from build123d import *

# Parameters (mm, degrees)
SKETCH_1_R               = 2.2
EXTRUDE_2_DEPTH          = 4
SKETCH_2_W               = 4
SKETCH_2_H               = 25
EXTRUDE_3_DEPTH          = 16
SKETCH_3_W               = 4
SKETCH_3_H               = 25
EXTRUDE_4_DEPTH          = 50
SKETCH_4_W               = 18
SKETCH_4_H               = 6.5
EXTRUDE_5_DEPTH          = 4
SKETCH_5_W               = 18
SKETCH_5_H               = 4
EXTRUDE_6_DEPTH          = 5
SKETCH_6_W               = 2.5
SKETCH_6_H               = 4
SKETCH_6_W_2             = 3
SKETCH_6_H_2             = 18
CUT_EXTRUDE_1_DEPTH      = 4
CUT_EXTRUDE_2_DEPTH      = 64.095166217
CUT_EXTRUDE_2_DEPTH_BACK = 64.095166217
SKETCH_7_R               = 4.7
CUT_EXTRUDE_3_DEPTH      = 64.095166217
EXTRUDE_7_DEPTH          = 3
EXTRUDE_8_DEPTH          = 3
CHAMFER_1_SIZE           = 3
CHAMFER_2_SIZE           = 2
FILLET_1_R               = 3
SKETCH_11_W              = 18
SKETCH_11_H              = 1
CUT_EXTRUDE_4_DEPTH      = 10
FILLET_2_R               = 2


with BuildPart() as part:
    # 草图1 → 凸台-拉伸2 (new body)
    with BuildSketch(Plane.XY):
        Polygon((0, 35), (0, 10), (-2.83, 10), (-2.83, 0), (9.32, 0), (9.32, 35), align=None)
        with Locations((2.17, 5)):
            Circle(SKETCH_1_R, mode=Mode.SUBTRACT)
        with Locations((5.17, 30)):
            Circle(SKETCH_1_R, mode=Mode.SUBTRACT)
    extrude(amount=EXTRUDE_2_DEPTH)

    # 草图2 → 凸台-拉伸3 (add)
    with BuildSketch(Plane(origin=(0, 0, 0), x_dir=(-1, 0, 0), z_dir=(0, 0, -1))):
        with Locations((2, 22.5)):
            Rectangle(SKETCH_2_W, SKETCH_2_H)
    extrude(amount=-EXTRUDE_3_DEPTH)

    # 草图3 → 凸台-拉伸4 (add)
    with BuildSketch(Plane(origin=(0, 0, 0), x_dir=(0, 0, -1), z_dir=(1, 0, 0))):
        with Locations((-14, 22.5)):
            Rectangle(SKETCH_3_W, SKETCH_3_H)
    extrude(amount=-EXTRUDE_4_DEPTH)

    # 草图4 → 凸台-拉伸5 (add)
    with BuildSketch(Plane(origin=(0, 0, 12), x_dir=(-1, 0, 0), z_dir=(0, 0, -1))):
        with Locations((33, 6.75)):
            Rectangle(SKETCH_4_W, SKETCH_4_H)
    extrude(amount=-EXTRUDE_5_DEPTH)

    # 草图5 → 凸台-拉伸6 (add)
    with BuildSketch(Plane(origin=(0, 0, 12), x_dir=(-1, 0, 0), z_dir=(0, 0, -1))):
        with Locations((33, 5.5)):
            Rectangle(SKETCH_5_W, SKETCH_5_H)
        with Locations((33, 33)):
            Rectangle(SKETCH_5_W, SKETCH_5_H)
    extrude(amount=EXTRUDE_6_DEPTH)

    # 草图6 → 切除-拉伸1 (cut)
    with BuildSketch(Plane(origin=(0, 0, 12), x_dir=(-1, 0, 0), z_dir=(0, 0, -1))):
        with Locations((15.05, 12)):
            Rectangle(SKETCH_6_W, SKETCH_6_H)
        with Locations((48.5, 19)):
            Rectangle(SKETCH_6_W_2, SKETCH_6_H_2)
    extrude(amount=-CUT_EXTRUDE_1_DEPTH, mode=Mode.SUBTRACT)

    # 草图7 → 切除-拉伸2 (cut, two sides: drawn at the far end of the back side and taken through both)
    with BuildSketch(Plane(origin=(0, 0, 0), x_dir=(0, 0, -1), z_dir=(1, 0, 0)).offset(-CUT_EXTRUDE_2_DEPTH_BACK)):
        with Locations(Location((-7.3, 20, 0), (0, 0, 45.402043339))):
            Circle(SKETCH_7_R)
    extrude(amount=CUT_EXTRUDE_2_DEPTH + CUT_EXTRUDE_2_DEPTH_BACK, mode=Mode.SUBTRACT)

    # 草图8 → 切除-拉伸3 (cut, through all)
    with BuildSketch(Plane(origin=(0, 0, 0), x_dir=(0, 0, -1), z_dir=(1, 0, 0))):
        with BuildLine():
            Line((-4, 24.274342055), (-4, 23.346640106))
            ThreePointArc((-4, 23.346640106), (-12, 20), (-4, 16.653359894))
            Line((-4, 16.653359894), (-4, 15.725657945))
            ThreePointArc((-4, 15.725657945), (-2.453351674, 17.61882382), (-1.9, 20))
            ThreePointArc((-1.9, 20), (-2.453351674, 22.38117618), (-4, 24.274342055))
        make_face()
        with BuildLine():
            ThreePointArc((-4, 16.653359894), (-12, 20), (-4, 23.346640106))
            Line((-4, 23.346640106), (-4, 24.274342055))
            ThreePointArc((-4, 24.274342055), (-12.7, 20), (-4, 15.725657945))
            Line((-4, 15.725657945), (-4, 16.653359894))
        make_face()
    extrude(amount=CUT_EXTRUDE_3_DEPTH, mode=Mode.SUBTRACT)

    # 草图9 → 凸台-拉伸7 (add)
    with BuildSketch(Plane.XZ.offset(-10)):
        Polygon((3.97, 4), (-0.03, 4), (0, 12), align=None)
        Polygon((-6, 12), (-4, 12), (-4, 7), align=None)
    extrude(amount=-EXTRUDE_7_DEPTH)

    # 草图10 → 凸台-拉伸8 (add)
    with BuildSketch(Plane(origin=(0, 35, 0), x_dir=(1, 0, 0), z_dir=(0, 1, 0))):
        Polygon((3.97, -4), (0, -4), (0, -12), align=None)
        Polygon((-4, -7), (-6, -12), (-4, -12), align=None)
    extrude(amount=-EXTRUDE_8_DEPTH)

    # 倒角1
    chamfer_1_edges = [part.edges().sort_by_distance(p)[0] for p in [
        (0, 22.5, 16),
        (-25, 35, 16),
        (-33, 3.5, 16),
    ]]
    chamfer(chamfer_1_edges, length=CHAMFER_1_SIZE)

    # 倒角2
    chamfer_2_edges = [part.edges().sort_by_distance(p)[0] for p in [
        (-13.8, 10, 14),
        (-16.3, 10, 14),
        (-50, 28, 14),
        (-47, 19, 12),
        (-50, 35, 12.5),
        (-33, 7.5, 7),
        (-33, 31, 7),
    ]]
    chamfer(chamfer_2_edges, length=CHAMFER_2_SIZE)

    # 圆角1
    fillet_1_edges = [part.edges().sort_by_distance(p)[0] for p in [
        (9.32, 35, 2),
        (9.32, 0, 2),
        (-2.83, 0, 2),
    ]]
    fillet(fillet_1_edges, radius=FILLET_1_R)

    # 草图11 → 切除-拉伸4 (cut)
    with BuildSketch(Plane(origin=(0, 0, 7), x_dir=(-1, 0, 0), z_dir=(0, 0, -1))):
        with Locations((33, 34.5)):
            Rectangle(SKETCH_11_W, SKETCH_11_H)
        with Locations((33, 4)):
            Rectangle(SKETCH_11_W, SKETCH_11_H)
    extrude(amount=-CUT_EXTRUDE_4_DEPTH, mode=Mode.SUBTRACT)

    # 圆角2
    fillet_2_edges = [part.edges().sort_by_distance(p)[0] for p in [
        (-33, 7.5, 12),
        (-33, 31, 12),
    ]]
    fillet(fillet_2_edges, radius=FILLET_2_R)


solid = part.part
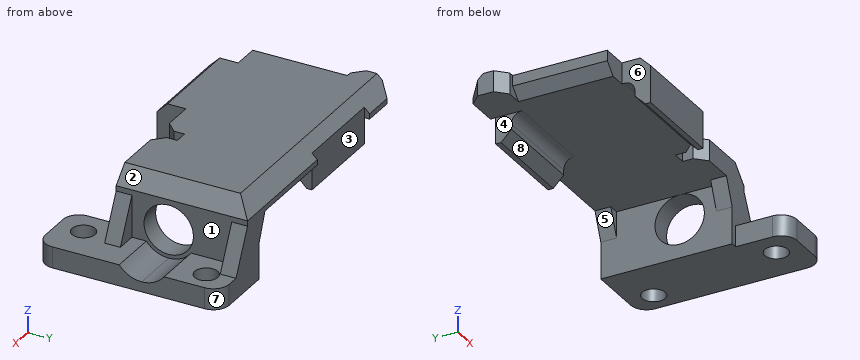
Geometry: final body of the model. Coordinates: model frame, mm. Face numbers are marked on the shaded views. A direction names the side the tool comes from. Round coordinates to 2 decimals unless told otherwise and drop trailing zeros. Loops run counter-clockwise (first coordinate to the right, second up) from the corner with the lowest first, then second, coordinate; pieces in that order, holes last.
Q1. Material intervals for L1, parallel to Y at x = -1.75, z = 7.3; L2, parallel to Y at x = 2.17, z = 2.7; L3, parallel to Y at x = 5.17, z = 1.8, sorted ascending.
Q2. Section C-C on x = -37. Return loops of the section in (y, z), plus the area to 3 significant figures.
Q3. Pull-direction query (Y, two-part tool) for the marked faces 6, 7 and 8; classes: released by +Y, released by -Y, zero draft, split by the parting line, or undercut.
Q4. Section B-B on z = 11. Return loops of the section in (x, y), plus the area to 3 significant figures.
Q5. Pin query (flat end, axial travel): P1, Ø4, axis at x = -5.5, y = 9.5, coming from the +Z side; P2, Ø2, axis at y = 31, z = 8.5, coming from the -X side; P3, Ø1.2, axis at y = 5, z = 2.5, coming from the -X side; P4, Ø1.6, axis at x = -5.5, z = 9.5, coming from the -Y side. Return the tip coordinate at first contact, or that it passes through.
Q6. Access query for the marked faces 1, 2, 3, 4 and 5. Directions: +Z, -Z, +X, -X, +Y, -Y. A direction counts if a zero-diameter tool reaches every point of the face in a straight line with its end or side. Return the directions, or none.
Q7. Section A-A on x = 5.17. Return loops of the section in (y, z), plus the area to 3 significant figures.
Evaluation:
1. L1: y = 10 to 15.3, 24.7 to 35
1. L2: y = 0 to 2.8, 7.2 to 17.17, 22.83 to 35
1. L3: y = 0 to 27.8, 32.2 to 35
2. outline: (4.5, 7) - (5.5, 7) - (7.5, 9) - (7.5, 10) arc R2 cw to (9.5, 12) - (29, 12) arc R2 cw to (31, 10) - (31, 9) - (33, 7) - (34, 7) - (34, 14) - (32, 16) - (6.5, 16) - (4.5, 14) - close
2. area: 142 mm2
3. face 6: zero draft
3. face 7: released by +Y
3. face 8: undercut
4. outline: (-42, 4.5) - (-24, 4.5) - (-24, 7.77) - (-42, 7.77) - close; (-42, 30.73) - (-24, 30.73) - (-24, 34) - (-42, 34) - close; (-5.6, 10) - (0.5, 10) - (0.5, 13) - (0, 13) - (0, 17.1) - (-4, 17.1) - (-4, 13) - (-5.6, 13) - close; (-5.6, 32) - (-4, 32) - (-4, 22.9) - (0, 22.9) - (0, 32) - (0.5, 32) - (0.5, 35) - (-5.6, 35) - close
4. area: 207 mm2
5. P1: stops at z = 16
5. P2: stops at x = -42
5. P3: stops at x = -2.83
5. P4: stops at y = 10
6. face 1: +Z, +X
6. face 2: +Z, +X, +Y, -Y
6. face 3: +Z, -Z, +Y
6. face 4: -Z, -X, +Y, -Y
6. face 5: -Z, +Y, -Y
7. outline: (0, 0) - (27.8, 0) - (27.8, 4) - (24.27, 4) arc R5.4 cw to (15.73, 4) - (0, 4) - close; (32.2, 0) - (35, 0) - (35, 4) - (32.2, 4) - close
7. area: 110 mm2
